Verification items for the finished model (mm, model axes). A direction names the side the tool comes from. Coordinates: 2 decimals unless noted, no trailing zeros. Loops run counter-clockwise (first coordinate to the right, second up) from the corner with the lowest first, then second, coordinate; pieces in that order, holes last. Notation, with made-up numbers: (1, 1.5) - (42, 1.5) arc R30 ccw to (42, 26.5) - close; hole circle Ø11 at (-35.75, 23.25). An arc over 180 degrees is marked (long way). Answer as CSV lines item,"result". Start each with the question number.
1. Material ranges on line 1 (Z direction, x = 5.2, y = 0.6); line 2 (Y direction, x = 0.45, z = 335); line 3 (Y direction, x = 9.25, z = 214), recorded low to high. Write a range as [from, to].
2. Cross-section at B-B (z = 282). Enter the section's corners in (x, y).
3. Gauge pin test, flat end, axial feed: P1, Ø4.5, axis at x = 5, z = 223.5, coming from the +Y side. Record the tip position at first contact, or that the pin passes through.
4. Set-up check for faces 1 (the flat face through (1, 6, 0)), 2 (the flat face through (1.2, 11, 168)): record each of +Z, -Z, +X, -X, +Y, -Y from which the full face is reachable in a straight line by a thin tool's end or side.
5. Cross-section at A-A (x = 5.2). Enter the section's corners in (y, z), plus the area to 3 significant figures.
6. Cross-section at C-C (y = 5.5). Enter the section's corners in (x, z).
```python
from build123d import *

# Parameters (mm, degrees)
EXTRUDE_1_DEPTH       = 340
HOLE_WIZARD_M41_D     = 4.5
HOLE_WIZARD_M41_DEPTH = 5
HOLE_WIZARD_M41_TIP   = 1.351936393
HOLE_WIZARD_M42_D     = 4.5
HOLE_WIZARD_M42_DEPTH = 5
HOLE_WIZARD_M42_TIP   = 1.351936393


with BuildPart() as part:
    # Эскиз1 → Бобышка-Вытянуть1 (new body)
    with BuildSketch(Plane.XY):
        Polygon((0, 0), (0, 20), (1.2, 20), (1.2, 1.2), (10, 1.2), (10, 0), align=None)
    extrude(amount=EXTRUDE_1_DEPTH)

    # Отверстие с зазором M41
    with Locations(Plane.ZY):
        with Locations((335, 11.2), (5, 11.2)):
            Hole(HOLE_WIZARD_M41_D / 2, depth=HOLE_WIZARD_M41_DEPTH)
            with Locations((0, 0, -(HOLE_WIZARD_M41_DEPTH + HOLE_WIZARD_M41_TIP / 2))):  # 118° drill point
                Cone(0, HOLE_WIZARD_M41_D / 2, HOLE_WIZARD_M41_TIP, mode=Mode.SUBTRACT)

    # Отверстие с зазором M42
    with Locations(Plane.XZ):
        with Locations((5.2, 5), (5.2, 335)):
            Hole(HOLE_WIZARD_M42_D / 2, depth=HOLE_WIZARD_M42_DEPTH)
            with Locations((0, 0, -(HOLE_WIZARD_M42_DEPTH + HOLE_WIZARD_M42_TIP / 2))):  # 118° drill point
                Cone(0, HOLE_WIZARD_M42_D / 2, HOLE_WIZARD_M42_TIP, mode=Mode.SUBTRACT)


solid = part.part
```
Values follow:
1,line 1,"z = [0, 2.75], [7.25, 332.75], [337.25, 340]"
1,line 2,"y = [0, 8.95], [13.45, 20]"
1,line 3,"y = [0, 1.2]"
2,outline,"(0, 0) - (10, 0) - (10, 1.2) - (1.2, 1.2) - (1.2, 20) - (0, 20) - close"
3,P1,"stops at y = 1.2"
4,face 1,"-Z, +X, -X, +Y, -Y"
4,face 2,"+Z, -Z, +X, +Y"
5,outline,"(0, 0) - (1.2, 0) - (1.2, 2.75) - (0, 2.75) - close; (0, 7.25) - (1.2, 7.25) - (1.2, 332.75) - (0, 332.75) - close; (0, 337.25) - (1.2, 337.25) - (1.2, 340) - (0, 340) - close"
5,area,"397 mm²"
6,outline,"(0, 0) - (1.2, 0) - (1.2, 340) - (0, 340) - close"
